The listing builds one solid part. Answer for the finished solid, in the listing's coordinates (mm). Round coordinates to 2 decimals unless told otherwise and drop trailing zeros. Order: outer loops, then holes, each group sorted by start corner. A loop starts at its lowest first (then second) coordinate and runs counter-clockwise, first axis right, second up. Notation, with made-up numbers: (-18, -38) - (14, -38) arc R22 ccw to (14, -8) - close; hole circle Ø4 at (41, 29.5). An arc over 180 degrees is marked (long way). One line per item, written item: value. Start each with the question number.
1. Section C-C, the plane x = -115 is taken. Give the vertices of the cut face in (y, z), then the cut area to 3 significant figures.
2. Straight lines are drawn through the part: line 1 (X direction, y = 0.6, z = 65); line 2 (Z direction, x = -111.5, y = 0.85); line 3 (X direction, y = 2.8, z = 20). For each, find the intervals that lie inside material, in ascending order.
3. Section B-B, the plane z = 35.5 is taken. Give the vertices of the cut face in (x, y).
4. Section A-A, the plane x = -132.5 is taken. Give the vertices of the cut face in (y, z).
5. Flat-ended cylindrical pins translate along their axes: P1, Ø2.5, axis at x = -61, z = 26.5, coming from the -Y side (3 decimals); P2, Ø0.9, axis at y = 2, z = 10.5, coming from the -X side. Find the tip coordinate at first contact, or state that the pin passes through.
6. Section D-D, the plane y = 1.05 is taken. Count the separate pieces of the cut face and the enclosed holes in it, then the cut area to 3 significant figures.
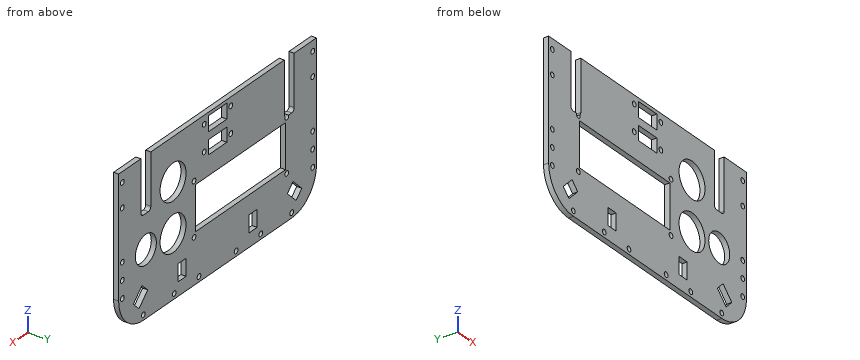
from build123d import *

# Parameters (mm, degrees)
CROQUIS1_R              = 1.5
CROQUIS1_R_2            = 10.5
CROQUIS1_R_3            = 8.5
CROQUIS1_W              = 73
CROQUIS1_H              = 26
CROQUIS1_W_2            = 6.5
CROQUIS1_H_2            = 10
SALIENTE_EXTRUIR2_DEPTH = 3
CORTAR_EXTRUIR1_DEPTH   = 10
CROQUIS3_R              = 1.5
CORTAR_EXTRUIR2_DEPTH   = 10
CROQUIS4_W              = 15
CROQUIS4_H              = 8.401372908
CROQUIS4_H_2            = 8.862986804
CORTAR_EXTRUIR3_DEPTH   = 10


with BuildPart() as part:
    # Croquis1 → Saliente-Extruir2 (new body)
    with BuildSketch(Plane(origin=(0, 0, 0), x_dir=(1, 0, 0), z_dir=(0, 1, 0))):
        with BuildLine():
            Line((-20, 0), (-140, 0))
            ThreePointArc((-140, 0), (-154.142135624, -5.857864376), (-160, -20))
            Line((-160, -20), (-160, -90))
            Line((-160, -90), (0, -90))
            Line((0, -90), (0, -20))
            ThreePointArc((0, -20), (-5.857864376, -5.857864376), (-20, 0))
        make_face()
        with Locations(Location((-61, -26.5, 0), (0, 0, 270))):
            Circle(CROQUIS1_R, mode=Mode.SUBTRACT)
        with Locations(Location((-61, -57.5, 0), (0, 0, 270))):
            Circle(CROQUIS1_R, mode=Mode.SUBTRACT)
        with Locations(Location((-136, -57.5, 0), (0, 0, 270))):
            Circle(CROQUIS1_R, mode=Mode.SUBTRACT)
        with Locations(Location((-136, -26.5, 0), (0, 0, 270))):
            Circle(CROQUIS1_R, mode=Mode.SUBTRACT)
        with Locations(Location((-44, -65, 0), (0, 0, 270))):
            Circle(CROQUIS1_R_2, mode=Mode.SUBTRACT)
        with Locations(Location((-44, -36.51645059, 0), (0, 0, 270))):
            Circle(CROQUIS1_R_2, mode=Mode.SUBTRACT)
        with Locations(Location((-22, -38, 0), (0, 0, 270))):
            Circle(CROQUIS1_R_3, mode=Mode.SUBTRACT)
        with Locations(Location((-90.795, -69.76, 0), (0, 0, 270))):
            Circle(CROQUIS1_R, mode=Mode.SUBTRACT)
        with Locations(Location((-69.205, -69.76, 0), (0, 0, 270))):
            Circle(CROQUIS1_R, mode=Mode.SUBTRACT)
        with Locations(Location((-69.205, -85, 0), (0, 0, 270))):
            Circle(CROQUIS1_R, mode=Mode.SUBTRACT)
        with Locations(Location((-90.795, -85, 0), (0, 0, 270))):
            Circle(CROQUIS1_R, mode=Mode.SUBTRACT)
        with Locations((-98.5, -42)):
            Rectangle(CROQUIS1_W, CROQUIS1_H, mode=Mode.SUBTRACT)
        Polygon((-148.16726189, -12.596194078), (-143.571067812, -8), (-136.5, -15.071067812), (-141.096194078, -19.66726189), align=None, mode=Mode.SUBTRACT)
        with Locations((-51.25, -13)):
            Rectangle(CROQUIS1_W_2, CROQUIS1_H_2, mode=Mode.SUBTRACT)
        with Locations((-108.75, -13)):
            Rectangle(CROQUIS1_W_2, CROQUIS1_H_2, mode=Mode.SUBTRACT)
        Polygon((-16.428932188, -8), (-11.83273811, -12.596194078), (-18.903805922, -19.66726189), (-23.5, -15.071067812), align=None, mode=Mode.SUBTRACT)
    extrude(amount=SALIENTE_EXTRUIR2_DEPTH)

    # Croquis2 → Cortar-Extruir1 (cut)
    with BuildSketch(Plane(origin=(0, 3, 0), x_dir=(1, 0, 0), z_dir=(0, 1, 0))):
        with BuildLine():
            Line((-142, -90), (-134, -90))
            Line((-134, -90), (-134, -60))
            ThreePointArc((-134, -60), (-134.585786438, -58.585786438), (-136, -58))
            Line((-136, -58), (-140, -58))
            ThreePointArc((-140, -58), (-141.414213562, -58.585786438), (-142, -60))
            Line((-142, -60), (-142, -90))
        make_face()
        with BuildLine():
            Line((-26, -90), (-18, -90))
            Line((-18, -90), (-18, -60))
            ThreePointArc((-18, -60), (-18.585786438, -58.585786438), (-20, -58))
            Line((-20, -58), (-24, -58))
            ThreePointArc((-24, -58), (-25.414213562, -58.585786438), (-26, -60))
            Line((-26, -60), (-26, -90))
        make_face()
    extrude(amount=-CORTAR_EXTRUIR1_DEPTH, mode=Mode.SUBTRACT)

    # Croquis3 → Cortar-Extruir2 (cut)
    with BuildSketch(Plane(origin=(0, 3, 0), x_dir=(1, 0, 0), z_dir=(0, 1, 0))):
        with Locations(Location((-157, -84, 0), (0, 0, 270))):
            Circle(CROQUIS3_R)
        with Locations(Location((-157, -70, 0), (0, 0, 270))):
            Circle(CROQUIS3_R)
        with Locations(Location((-157, -40, 0), (0, 0, 270))):
            Circle(CROQUIS3_R)
        with Locations(Location((-157, -30, 0), (0, 0, 270))):
            Circle(CROQUIS3_R)
        with Locations(Location((-140, -3, 0), (0, 0, 270))):
            Circle(CROQUIS3_R)
        with Locations(Location((-115, -3, 0), (0, 0, 270))):
            Circle(CROQUIS3_R)
        with Locations(Location((-95, -3, 0), (0, 0, 270))):
            Circle(CROQUIS3_R)
        with Locations(Location((-65, -3, 0), (0, 0, 270))):
            Circle(CROQUIS3_R)
        with Locations(Location((-45, -3, 0), (0, 0, 270))):
            Circle(CROQUIS3_R)
        with Locations(Location((-20, -3, 0), (0, 0, 270))):
            Circle(CROQUIS3_R)
        with Locations(Location((-3, -30, 0), (0, 0, 270))):
            Circle(CROQUIS3_R)
        with Locations(Location((-3, -40, 0), (0, 0, 270))):
            Circle(CROQUIS3_R)
        with Locations(Location((-3, -70, 0), (0, 0, 270))):
            Circle(CROQUIS3_R)
        with Locations(Location((-3, -84, 0), (0, 0, 270))):
            Circle(CROQUIS3_R)
        with Locations(Location((-157, -20, 0), (0, 0, 270))):
            Circle(CROQUIS3_R)
        with Locations(Location((-3, -20, 0), (0, 0, 270))):
            Circle(CROQUIS3_R)
    extrude(amount=-CORTAR_EXTRUIR2_DEPTH, mode=Mode.SUBTRACT)

    # Croquis4 → Cortar-Extruir3 (cut)
    with BuildSketch(Plane(origin=(0, 3, 0), x_dir=(1, 0, 0), z_dir=(0, 1, 0))):
        with Locations((-80, -70.663029374)):
            Rectangle(CROQUIS4_W, CROQUIS4_H)
        with Locations((-80, -83.634379853)):
            Rectangle(CROQUIS4_W, CROQUIS4_H_2)
    extrude(amount=-CORTAR_EXTRUIR3_DEPTH, mode=Mode.SUBTRACT)


solid = part.part
Answer list:
1. outline: (0, 0) - (3, 0) - (3, 1.5) - (0, 1.5) - close; (0, 4.5) - (3, 4.5) - (3, 29) - (0, 29) - close; (0, 55) - (3, 55) - (3, 90) - (0, 90) - close
1. area: 183 mm²
2. line 1: x = -160 to -142, -134 to -54.5, -33.5 to -26, -18 to 0
2. line 2: z = 0 to 8, 18 to 29, 55 to 90
2. line 3: x = -160 to -158.5, -155.5 to -4.5, -1.5 to 0
3. outline: (-160, 0) - (-135, 0) - (-135, 3) - (-160, 3) - close; (-62, 0) - (-54.45, 0) - (-54.45, 3) - (-62, 3) - close; (-33.55, 0) - (-30.12, 0) - (-30.12, 3) - (-33.55, 3) - close; (-13.88, 0) - (0, 0) - (0, 3) - (-13.88, 3) - close
4. outline: (0, 0) - (3, 0) - (3, 29) - (0, 29) - close; (0, 55) - (3, 55) - (3, 90) - (0, 90) - close
5. P1: passes through
5. P2: stops at x = -157.84
6. separate pieces: 1
6. enclosed holes: 33
6. area: 10,200 mm²
